Work out the finished part from the listing and answer in its coordinate system (mm). A direction names the side the tool comes from. Coordinates: 2 decimals unless noted, no trailing zeros. Write each loop counter-clockwise with the first axis right and the second up, starting at its lowest first coordinate (ties: lowest second). Pieces come first, ordered by that corner, then holes. Notation, with made-up numbers: M 36.25,14 L 83.25,14 A17 cw 83.25,35 Z; hole C 79.5,5 d9. An arc over 180 degrees is marked long. Use CSV: the item, a comma, the result in double quotes.
from build123d import *

# Parameters (mm, degrees)
F1_DEPTH = 71.4375
F2_R     = 1.9812
F3_DEPTH = 6.096
F4_R     = 1.9812
F5_DEPTH = 6.096


with BuildPart() as f1:
    # F0 (on Front) → F1 (new body)
    with BuildSketch(Plane.XZ):
        Polygon((3.181334, 6.092442), (3.181334, 12.188442), (-2.914666, 12.188442), (-2.914666, -1.273558), (28.327334, -1.273558), (28.327334, 12.188442), (22.231334, 12.188442), (22.231334, 6.092442), (24.390334, 6.092442), (24.390334, 2.536442), (1.022334, 2.536442), (1.022334, 6.092442), align=None)
    extrude(amount=F1_DEPTH)

    # F2 (on face) → F3 (cut, through all)
    with BuildSketch(Plane.YZ.offset(28.327334)):
        with Locations((-13.335, 8.759442)):
            Circle(F2_R)
    extrude(amount=-F3_DEPTH, mode=Mode.SUBTRACT)

    # F4 (on face) → F5 (cut, through all)
    with BuildSketch(Plane(origin=(-2.914666, 0, 0), x_dir=(0, -1, 0), z_dir=(-1, 0, 0))):
        with Locations((13.335, 8.759442)):
            Circle(F4_R)
    extrude(amount=-F5_DEPTH, mode=Mode.SUBTRACT)


solid = f1.part
Item 1: The part is cut by section B-B (z = 5). Write down the section's boundary in (x, y), then the cut area to 4 significant figures.
Answer:
outline,"M -2.91,-71.44 L 1.02,-71.44 L 1.02,0 L -2.91,0 Z; M 24.39,-71.44 L 28.33,-71.44 L 28.33,0 L 24.39,0 Z"
area,"562.5 mm2"
Item 2: A tool of negligible diameter and unlimited length cuts with its end or side. For faces 1 (the face through (22.231, -35, 9)), 2 (the face through (24.39, -35, 4)), 3 (the face through (0, -35, 12.188)), from which of +Z, -Z, +X, -X, +Y, -Y can it reach the whole face along a straight path? Write none if from no direction.
Answer:
face 1,"+Z, +Y, -Y"
face 2,"+Y, -Y"
face 3,"+Z, +X, -X, +Y, -Y"
Item 3: For a pull along X with two mould halves and no side action, classify faces 4 (the face through (3.181, -35, 9)), 5 (the face through (25, -35, 12.188)), 6 (the face through (28.327, -35, 5)), 7 (the face through (13, -35, 2.536)) as released by +X, released by -X, zero draft, split by the parting line, or undercut.
Answer:
face 4,"undercut"
face 5,"zero draft"
face 6,"released by +X"
face 7,"undercut"
Item 4: Given pin 1 (7 mm diameter, centred on x = 7.5, y = -51, fed in from +Z); pin 2 (1.5 mm diameter, centred on x = 24, z = 4, fed in from +Y), each flat-ended and moving along its own axis, determine where each tip first touches the part or whether it passes through.
Answer:
pin 1,"stops at z = 2.54"
pin 2,"stops at y = 0"
Item 5: The part is cut by section D-D (y = -10). Write down the section's boundary in (x, z).
Answer:
outline,"M -2.91,-1.27 L 28.33,-1.27 L 28.33,12.19 L 22.23,12.19 L 22.23,6.09 L 24.39,6.09 L 24.39,2.54 L 1.02,2.54 L 1.02,6.09 L 3.18,6.09 L 3.18,12.19 L -2.91,12.19 Z"
Item 6: The part is cut by section A-A (x = 23.5). Write down the section's boundary in (y, z) (1 decimal), then the cut area to 3 significant figures.
Answer:
outline,"M -71.4,-1.3 L 0,-1.3 L 0,2.5 L -71.4,2.5 Z; M -71.4,6.1 L 0,6.1 L 0,12.2 L -71.4,12.2 Z; hole C -13.3,8.8 d4"
area,"695 mm2"
Item 7: Consider probe 1 along X at (y, z) = (-15.5, 2.75); probe 2 along X at (y, z) = (-55, 6.5); probe 3 along Z at (x, y) = (22.5, -45.5). Determine where each line is inside the solid, lowest interval first.
Answer:
probe 1,"x = -2.91 to 1.02, 24.39 to 28.33"
probe 2,"x = -2.91 to 3.18, 22.23 to 28.33"
probe 3,"z = -1.27 to 2.54, 6.09 to 12.19"
Item 8: The part is cut by section C-C (z = 10). Write down the section's boundary in (x, y).
Answer:
outline,"M -2.91,-71.44 L 3.18,-71.44 L 3.18,-14.88 L -2.91,-14.88 Z; M -2.91,-11.79 L 3.18,-11.79 L 3.18,0 L -2.91,0 Z; M 22.23,-71.44 L 28.33,-71.44 L 28.33,-14.88 L 22.23,-14.88 Z; M 22.23,-11.79 L 28.33,-11.79 L 28.33,0 L 22.23,0 Z"
